Input: part model. Units: mm. Frame: model coordinates. A direction names the side the tool comes from. Coordinates: 2 decimals unless noted, no trailing zeros. Loops run counter-clockwise (first coordinate to the right, second up) from the corner with the lowest first, then second, coordinate; pieces in that order, holes last.
Autodesk Inventor part; units mm, degrees
ref_plane "YZ Plane" through (0, 0, 0) normal (1, 0, 0) x (0, 1, 0)
ref_plane "XZ Plane" through (0, 0, 0) normal (0, 1, 0) x (-1, 0, 0)
ref_plane "XY Plane" through (0, 0, 0) normal (0, 0, 1) x (1, 0, 0)
sketch "Sketch1" plane through (0, 0, 0) normal (0, 0, 1) x (1, 0, 0)
  line L0 (-40, 12.5) -> (40, 12.5)
  line L1 (40, 12.5) -> (40, -12.5)
  line L2 (40, -12.5) -> (-40, -12.5)
  line L3 (-40, -12.5) -> (-40, 12.5)
  circle A0 centre (-30, 0) radius 2.15
  circle A1 centre (-5, 0) radius 2.15
  circle A2 centre (5, 0) radius 2.15
  circle A3 centre (30, 0) radius 2.15
  point P0 (0, 0)
  point P1 (0, 12.5)
  point P2 (-40, 0)
  dimension "d0" = 25
  dimension "d1" = 80
  dimension "d9" = 4.3
  dimension "d10" = 5
  dimension "d11" = 5
  dimension "d12" = 10
  dimension "d13" = 10
extrude "Extrusion1" add sketch "Sketch1" along normal blind 3
sketch "Sketch2" plane through (0, 0, 3) normal (0, 0, 1) x (1, 0, 0)
  line L0 (-40, -12.5) -> (40, -12.5)
  line L1 (40, -12.5) -> (40, 12.5)
  line L2 (40, 12.5) -> (-40, 12.5)
  line L3 (-40, 12.5) -> (-40, -12.5)
  line L4 (-40, 12.5) -> (-40, -12.5)
  line L5 (-40, 10) -> (40, 10)
  line L6 (40, -12.5) -> (40, 12.5)
  line L7 (40, -12.5) -> (40, 12.5)
  line L8 (40, -10) -> (-40, -10)
  point P0 (0, 0)
  dimension "d4" = 2.5
  dimension "d5" = 2.5
  dimension "d6" = 20
extrude "Extrusion2" add sketch "Sketch2" along normal blind 20 contours L3 L8 L1 L0 | L3 L2 L1 L5
equation "\"d12\" = 2 * d10"
equation "\"d13\" = d12"
equation "\"d5\" = d4"
properties part number "Verbinder"
Item 1: Section query B-B (y = 0). Output: boundary loops of the cut face in (x, z).
Result:
outline: (-40, 0) - (-32.15, 0) - (-32.15, 3) - (-40, 3) - close; (-27.85, 0) - (-7.15, 0) - (-7.15, 3) - (-27.85, 3) - close; (-2.85, 0) - (2.85, 0) - (2.85, 3) - (-2.85, 3) - close; (7.15, 0) - (27.85, 0) - (27.85, 3) - (7.15, 3) - close; (32.15, 0) - (40, 0) - (40, 3) - (32.15, 3) - close
Item 2: Contact query for flat-ended pins moving along their axis: P1, Ø6, axis at x = -19, y = 4, coming from the +Z side; P2, Ø12, axis at y = -1.5, z = 19, coming from the -X side; P3, Ø10, axis at x = 21.5, y = 3, coming from the -Z side. Output: stop coordinate, or through.
Result:
P1: stops at z = 3
P2: passes through
P3: stops at z = 0
Item 3: Section query A-A (z = 3.75). Output: boundary loops of the cut face in (x, y).
Result:
outline: (-40, -12.5) - (40, -12.5) - (40, -10) - (-40, -10) - close; (-40, 10) - (40, 10) - (40, 12.5) - (-40, 12.5) - close
Item 4: Line query: L1, parallel to Y at x = 30, z = 2.2; L2, parallel to Y at x = -7.5, z = 17.25; L3, parallel to Z at x = 30, y = -9.25. Output: solid intervals per line, ascending.
Result:
L1: y = -12.5 to -2.15, 2.15 to 12.5
L2: y = -12.5 to -10, 10 to 12.5
L3: z = 0 to 3
Item 5: Section query D-D (y = -8.75). Output: boundary loops of the cut face in (x, z), then the cut area to 3 significant figures.
Result:
outline: (-40, 0) - (40, 0) - (40, 3) - (-40, 3) - close
area: 240 mm2
Item 6: Section query C-C (x = 5). Output: boundary loops of the cut face in (y, z).
Result:
outline: (-12.5, 0) - (-2.15, 0) - (-2.15, 3) - (-10, 3) - (-10, 23) - (-12.5, 23) - close; (2.15, 0) - (12.5, 0) - (12.5, 23) - (10, 23) - (10, 3) - (2.15, 3) - close
Item 7: Reachability of faces 1 (the face through (-1, 0, 0)), 2 (the face through (-1, 0, 3)) from +Z, -Z, +X, -X, +Y, -Y: full face, straight path, thin tool, end or side. Return the list, or none.
Result:
face 1: -Z, +X, -X, +Y, -Y
face 2: +Z, +X, -X
Item 8: Mould query, pull axis X, two halves, no side actions, for faces 3 (the face through (-7.15, -0.09, 1.48)), 4 (the face through (40, 1, 2)), 5 (the face through (-1, 12.5, 11)). Classes: +X half, -X half, draft (parallel to the pull), parting line (faces both ways), or undercut.
Result:
face 3: undercut
face 4: +X half
face 5: draft
